The listing builds one solid part. Answer for the finished solid, in the listing's coordinates (mm). A direction names the side the tool comes from. Give positions to 0.01 mm unless a question says otherwise; leave off trailing zeros. Loops run counter-clockwise (first coordinate to the right, second up) from the corner with the lowest first, then second, coordinate; pieces in that order, holes last. Notation, with made-up numbers: M -36.5,-22.75 L 4.5,-22.75 A7 cw 4.5,-12.75 Z; hole C 24,36.5 d9. An arc over 180 degrees is marked long. One line per item, written item: value. Start each with the question number.
Q1. Flat-ended cylindrical pins translate along their axes: pin 1 (1 mm diameter, centred on y = 2, z = 3, fed in from +X); pin 2 (1.5 mm diameter, centred on y = 4, z = -6.5, fed in from -X); pin 3 (1.5 mm diameter, centred on x = 0, y = 2.5, fed in from -Z). Find the tip coordinate at first contact, or state that the pin passes through.
Q2. A cutting plane is placed at C-C, the plane y = 2.5. Determine the outline of the cut face in (x, z) (3 decimals), and give its area (3 significant figures).
Q3. A cutting plane is placed at A-A, the plane x = 0. Determine the outline of the cut face in (y, z) (3 decimals), and give its area (3 significant figures).
Q4. A cutting plane is placed at B-B, the plane z = 3.75. Determine the outline of the cut face in (x, y), and give its area (3 significant figures).
Q5. The mould has two halves that part along X. Classify faces 1 (the cylindrical face through (4.38, 2.46, 8.43)), 2 (the cylindrical face through (-3.13, 2.46, 4.06)), 3 (the flat face through (-0.1, 5, -2.2)): +X half, -X half, draft (parallel to the pull), parting line (faces both ways), or undercut.
Q6. A cutting plane is placed at D-D, the plane y = 0.75. Determine the outline of the cut face in (x, z) (3 decimals).
Q7. For faces 4 (the flat face through (-0.1, 0, -2.2)), 5 (the cylindrical face through (0.266, 1.304, -5.596)), determine the directions among +Z, -Z, +X, -X, +Y, -Y from which every point of the face is accessible in a straight line to the end or side of a thin tool.
Q8. Consider L1, parallel to X at y = 2.1, z = 0; L2, parallel to X at y = 4.4, z = 4.75; L3, parallel to Z at x = -3.5, y = 3.85. Determine where each line is inside the solid, lowest interval first.
from build123d import *

# Parameters (mm, degrees)
SKETCH1_R           = 9.5
SKETCH1_R_2         = 2
SKETCH1_R_3         = 1.425
BOSS_EXTRUDE1_DEPTH = 5
CUT_EXTRUDE1_REACH  = 21
SKETCH2_R           = 1.225


with BuildPart() as part:
    # Sketch1 → Boss-Extrude1 (new body)
    with BuildSketch(Plane(origin=(0, 0, 0), x_dir=(1, 0, 0), z_dir=(0, 1, 0))):
        Circle(SKETCH1_R)
        Circle(SKETCH1_R_2, mode=Mode.SUBTRACT)
        with Locations((-4.490128061, 4.490128061)):
            Circle(SKETCH1_R_3, mode=Mode.SUBTRACT)
        with Locations((4.490128061, 4.490128061)):
            Circle(SKETCH1_R_3, mode=Mode.SUBTRACT)
        with Locations((4.490128061, -4.490128061)):
            Circle(SKETCH1_R_3, mode=Mode.SUBTRACT)
        with Locations((-4.490128061, -4.490128061)):
            Circle(SKETCH1_R_3, mode=Mode.SUBTRACT)
    extrude(amount=BOSS_EXTRUDE1_DEPTH)

    # Sketch2 → Cut-Extrude1 (cut, up to next)
    with BuildSketch(Plane(origin=(0, 0, -9.5), x_dir=(-1, 0, 0), z_dir=(0, 0, -1)), mode=Mode.PRIVATE) as cut_extrude1_sk1:
        with Locations((0, 2.5)):
            Circle(SKETCH2_R)
    cut_extrude1_tool1 = extrude(cut_extrude1_sk1.sketch, amount=-CUT_EXTRUDE1_REACH, mode=Mode.PRIVATE) & part.part
    add(cut_extrude1_tool1.solids().sort_by_distance((0, 2.5, -9.5))[0], mode=Mode.SUBTRACT)


solid = part.part
Answer block:
1. pin 1: x = 9.17
1. pin 2: x = -7.56
1. pin 3: z = 1.85
2. outline: M -1.225,-9.421 L -1.225,-1.581 A2 cw long 1.225,-1.581 L 1.225,-9.421 A9.5 ccw long Z; hole C -4.49,-4.49 d2.85; hole C -4.49,4.49 d2.85; hole C 4.49,-4.49 d2.85; hole C 4.49,4.49 d2.85
2. area: 227 mm^2
3. outline: M 0,-9.5 L 1.275,-9.5 L 1.275,-2 L 0,-2 Z; M 0,2 L 5,2 L 5,9.5 L 0,9.5 Z; M 3.725,-9.5 L 5,-9.5 L 5,-2 L 3.725,-2 Z
3. area: 56.6 mm^2
4. outline: M -8.73,0 L -5.71,0 L -5.71,5 L -8.73,5 Z; M -3.27,0 L 3.27,0 L 3.27,5 L -3.27,5 Z; M 5.71,0 L 8.73,0 L 8.73,5 L 5.71,5 Z
4. area: 62.9 mm^2
5. face 1: parting line
5. face 2: undercut
5. face 3: draft
6. outline: C 0,0 d19; hole C -4.49,-4.49 d2.85; hole C -4.49,4.49 d2.85; hole C 0,0 d4; hole C 4.49,-4.49 d2.85; hole C 4.49,4.49 d2.85
7. face 4: +Z, -Z, +X, -X, -Y
7. face 5: -Z
8. L1: -9.5 to -2, 2 to 9.5
8. L2: -8.23 to -5.89, -3.09 to 3.09, 5.89 to 8.23
8. L3: -8.83 to -5.51, -3.47 to 3.47, 5.51 to 8.83
